```python
from build123d import *

# Parameters (mm, degrees)
CUT_EXTRUDE1_DEPTH = 15
CUT_EXTRUDE2_START = -40
SKETCH3_R          = 20
SKETCH3_R_2        = 18.5
CUT_EXTRUDE2_DEPTH = 1


with BuildPart() as part:
    # Sketch1 → Revolve1 (revolve)
    with BuildSketch(Plane(origin=(0, 0, 0), x_dir=(0, 0, -1), z_dir=(1, 0, 0)), mode=Mode.PRIVATE) as revolve1_sk:
        Polygon((0, 0), (0, 20), (100, 20), (100, 8), (120, 8), (120, 0), align=None)
    revolve(revolve1_sk.sketch.rotate(Axis((0, 0, 24.465289117), (0, 0, -1)), 90), axis=Axis((0, 0, 24.465289117), (0, 0, -1)))

    # Sketch2 → Cut-Extrude1 (cut)
    with BuildSketch(Plane(origin=(0, 0, -120), x_dir=(-1, 0, 0), z_dir=(0, 0, -1))):
        with BuildLine():
            Line((-6.92820323, 4), (6.92820323, 4))
            ThreePointArc((6.92820323, 4), (0, 8), (-6.92820323, 4))
        make_face()
    extrude(amount=-CUT_EXTRUDE1_DEPTH, mode=Mode.SUBTRACT)

    # Sketch3 → Cut-Extrude2 (cut)
    with BuildSketch(Plane(origin=(0, 0, -100), x_dir=(-1, 0, 0), z_dir=(0, 0, -1)).offset(CUT_EXTRUDE2_START)):
        with Locations(Location((0, 0, 0), (0, 0, 180))):
            Circle(SKETCH3_R)
        Circle(SKETCH3_R_2, mode=Mode.SUBTRACT)
    extrude(amount=-CUT_EXTRUDE2_DEPTH, mode=Mode.SUBTRACT)


solid = part.part
```
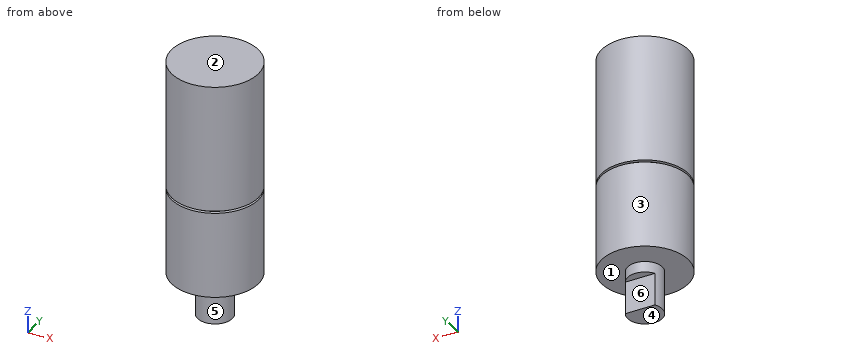
Verification items for the finished model (mm, model axes). Face numbers are marked on the shaded views. A direction names the side the tool comes from. Coordinates: 2 decimals unless noted, no trailing zeros. Order: outer loops, then holes, each group sorted by start corner. A loop starts at its lowest first (then second) coordinate and runs counter-clockwise, first axis right, second up. Notation, with made-up numbers: (-2.75, 71.5) -> (16.25, 71.5) arc R25 ccw to (16.25, 91.5) -> close; hole circle Ø8 at (45, 26). An arc over 180 degrees is marked (long way). Answer as CSV lines item,"result". Start each with the question number.
1) Cross-section at D-D, the plane y = -16. Record the boundary of the cut face in (x, z), then the cut area to 3 significant figures.
2) Release check for a two-part mould opening along Z. For the marked faces 1, 2 and 3 record: released by +Z, released by -Z, zero draft, split by the parting line, or undercut.
3) Gauge pin test, flat ends, axial feed: pin 1 Ø3 at (x, z) = (-6.5, -32) entering from +Y; pin 2 Ø15 at (x, z) = (1, -113.5) entering from +Y; pin 3 Ø4 at (x, z) = (-2.5, -43.5) entering from -Y; pin 4 Ø2 at (x, z) = (12, -102) entering from -Y. Record the tip position at first contact, or that the pin passes through.
4) Cross-section at B-B, the plane y = 0. Record the boundary of the cut face in (x, z).
5) Cross-section at A-A, the plane x = 0. Record the boundary of the cut face in (y, z).
6) Material ranges on L1, parallel to Z at x = -11, y = -6; L2, parallel to X at y = -1, z = -71; L3, parallel to Y at x = -0.5, z = -46.5, recorded low to high. Write a range as [from, to].
7) Cross-section at C-C, the plane z = -29. Record the boundary of the cut face in (x, y), then the cut area to 3 significant figures.
8) Set-up check for the marked faces 4, 5 and 6: record each of +Z, -Z, +X, -X, +Y, -Y from which the full face is reachable in a straight line by a thin tool's end or side.
Conclusion:
1,outline,"(-12, -100) -> (12, -100) -> (12, -60) -> (9.29, -60) -> (9.29, -59) -> (12, -59) -> (12, 0) -> (-12, 0) -> (-12, -59) -> (-9.29, -59) -> (-9.29, -60) -> (-12, -60) -> close"
1,area,"2,390 mm²"
2,face 1,"released by -Z"
2,face 2,"released by +Z"
2,face 3,"zero draft"
3,pin 1,"stops at y = 19.36"
3,pin 2,"stops at y = 4"
3,pin 3,"stops at y = -19.99"
3,pin 4,"passes through"
4,outline,"(-20, -100) -> (-8, -100) -> (-8, -120) -> (8, -120) -> (8, -100) -> (20, -100) -> (20, -60) -> (18.5, -60) -> (18.5, -59) -> (20, -59) -> (20, 0) -> (-20, 0) -> (-20, -59) -> (-18.5, -59) -> (-18.5, -60) -> (-20, -60) -> close"
5,outline,"(-20, -100) -> (-8, -100) -> (-8, -120) -> (4, -120) -> (4, -105) -> (8, -105) -> (8, -100) -> (20, -100) -> (20, -60) -> (18.5, -60) -> (18.5, -59) -> (20, -59) -> (20, 0) -> (-20, 0) -> (-20, -59) -> (-18.5, -59) -> (-18.5, -60) -> (-20, -60) -> close"
6,L1,"z = [-100, 0]"
6,L2,"x = [-19.97, 19.97]"
6,L3,"y = [-19.99, 19.99]"
7,outline,"circle Ø40 at (0, 0)"
7,area,"1,260 mm²"
8,face 4,"-Z, +X, -X, +Y, -Y"
8,face 5,"-Z"
8,face 6,"-Z, +X, -X, +Y"
